Design review of the part built by this model. Coordinates are the model's own, in mm. Give positions to 0.01 mm unless a question says otherwise; leave off trailing zeros. Write each loop counter-clockwise with the first axis right and the second up, starting at its lowest first coordinate (ties: lowest second). Pieces come first, ordered by that corner, then holes. Notation, with made-up numbers: M 74.5,-27 L 119.5,-27 A21 ccw 119.5,3 Z; hole C 10,45.5 d2. An arc over 180 degrees is marked long. Use one line per item in the form item = value. Start each with the question number.
from build123d import *

# Parameters (mm, degrees)
SKETCH1_R           = 140
SKETCH1_R_2         = 4.1
SKETCH1_R_3         = 106
BOSS_EXTRUDE1_DEPTH = 8
CHAMFER2_SIZE       = 1


with BuildPart() as part:
    # Sketch1 → Boss-Extrude1 (new body)
    with BuildSketch(Plane(origin=(0, 0, -8), x_dir=(-1, 0, 0), z_dir=(0, 0, -1))):
        with Locations(Location((0, 0, 0), (0, 0, 180))):
            Circle(SKETCH1_R)
        with Locations(Location((91.960251276, 91.887497437, 0), (0, 0, 180))):
            Circle(SKETCH1_R_2, mode=Mode.SUBTRACT)
        with Locations(Location((129.999989821, -0.051444733, 0), (0, 0, 180))):
            Circle(SKETCH1_R_2, mode=Mode.SUBTRACT)
        with Locations(Location((91.887497437, -91.960251276, 0), (0, 0, 180))):
            Circle(SKETCH1_R_2, mode=Mode.SUBTRACT)
        with Locations(Location((-0.051444733, -129.999989821, 0), (0, 0, 180))):
            Circle(SKETCH1_R_2, mode=Mode.SUBTRACT)
        with Locations(Location((-91.960251276, -91.887497437, 0), (0, 0, 180))):
            Circle(SKETCH1_R_2, mode=Mode.SUBTRACT)
        with Locations(Location((-129.999989821, 0.051444733, 0), (0, 0, 180))):
            Circle(SKETCH1_R_2, mode=Mode.SUBTRACT)
        with Locations(Location((-91.887497437, 91.960251276, 0), (0, 0, 180))):
            Circle(SKETCH1_R_2, mode=Mode.SUBTRACT)
        with Locations(Location((0.051444733, 129.999989821, 0), (0, 0, 180))):
            Circle(SKETCH1_R_2, mode=Mode.SUBTRACT)
        with Locations(Location((0, 0, 0), (0, 0, 180))):
            Circle(SKETCH1_R_3, mode=Mode.SUBTRACT)
    extrude(amount=-BOSS_EXTRUDE1_DEPTH)

    # Chamfer2
    chamfer2_edges = [part.edges().sort_by_distance(p)[0] for p in [
        (-140, 0, -8),
        (-106, 0, 0),
        (-106, 0, -8),
        (-140, 0, 0),
    ]]
    chamfer(chamfer2_edges, length=CHAMFER2_SIZE)


solid = part.part
1. We need section A-A (x = 0). State the section outline as (y, z) points, and give its area (3 significant figures).
2. To check wall thickness, follow L1, parallel to X at y = -92, z = -6.75; L2, parallel to X at y = -95, z = -5; L3, parallel to X at y = -25, z = -2.25. State the ranges of each line that lie inside material, in increasing order.
3. Clearance check with flat-ended pins moving along their axes: pin 1 Ø9.5 at (x, y) = (-91.89, -91.96) entering from +Z; pin 2 Ø2 at (y, z) = (98, -3) entering from +X; pin 3 Ø1 at (x, z) = (12.5, -1.5) entering from -Y. State where each tip first meets the part, or that it passes through.
4. Draft analysis for pull direction X (two halves, no side actions). For faces 1 (the flat face through (-73, 82, -8)), 2 (the cylindrical face through (-94.982, 89.117, -4.056)), 3 (the cylindrical face through (1.84, 133.637, -4.056)), 4 (the cylindrical face through (-30.35, 136.67, -4.04)), state which applies: pulls with the +X half, pulls with the -X half, needs draft (parallel to the pull), parting line crosses it, or undercut.
Answer block:
q1.outline = M -140,-7 L -139,-8 L -134.1,-8 L -134.1,0 L -139,0 L -140,-1 Z; M -125.9,-8 L -107,-8 L -106,-7 L -106,-1 L -107,0 L -125.9,0 Z; M 106,-7 L 107,-8 L 125.9,-8 L 125.9,0 L 107,0 L 106,-1 Z; M 134.1,-8 L 139,-8 L 140,-7 L 140,-1 L 139,0 L 134.1,0 Z
q1.area = 409 mm^2
q2.L1 = -105.53 to -95.99, -87.79 to -52.65, 52.65 to 87.86, 96.06 to 105.53
q2.L2 = -102.83 to -94.64, -89.14 to -47.02, 47.02 to 89.29, 94.63 to 102.83
q2.L3 = -137.75 to -103.01, 103.01 to 137.75
q3.pin_1 = 0
q3.pin_2 = 100.95
q3.pin_3 = -139.48
q4.face_1 = needs draft
q4.face_2 = undercut
q4.face_3 = undercut
q4.face_4 = parting line crosses it
